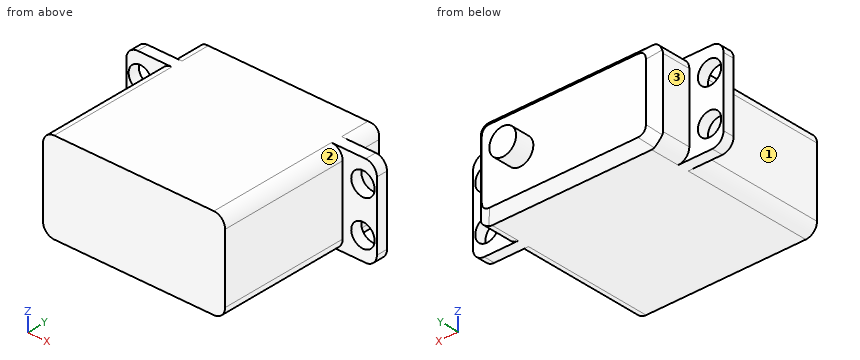
from build123d import *

# Parameters (mm, degrees)
BOSS_EXTRUDE1_DEPTH = 20.2
SKETCH2_R           = 2.975
BOSS_EXTRUDE2_DEPTH = 4.25
CUT_EXTRUDE1_START  = 29
SKETCH3_R           = 2.6
CUT_EXTRUDE1_DEPTH  = 4.25
CHAMFER1_SIZE       = 2
FILLET1_R           = 2.5


with BuildPart() as part:
    # Sketch1 → Boss-Extrude1 (new body)
    with BuildSketch(Plane.XY):
        Polygon((-20.25, 0), (20.25, 0), (20.25, 29), (27.85, 29), (27.85, 31.5), (20.25, 31.5), (20.25, 40), (-20.25, 40), (-20.25, 31.5), (-27.85, 31.5), (-27.85, 29), (-20.25, 29), align=None)
    extrude(amount=BOSS_EXTRUDE1_DEPTH)

    # Sketch2 → Boss-Extrude2 (add)
    with BuildSketch(Plane(origin=(0, 40, 0), x_dir=(1, 0, 0), z_dir=(0, 1, 0))):
        with Locations(Location((9.75, -10.1, 0), (0, 0, 90))):
            Circle(SKETCH2_R)
    extrude(amount=BOSS_EXTRUDE2_DEPTH)

    # Sketch3 → Cut-Extrude1 (cut)
    with BuildSketch(Plane(origin=(0, 0, 0), x_dir=(1, 0, 0), z_dir=(0, 1, 0)).offset(CUT_EXTRUDE1_START)):
        with Locations(Location((-24.75, -5.1, 0), (0, 0, 90))):
            Circle(SKETCH3_R)
        with Locations(Location((-24.75, -15.1, 0), (0, 0, 90))):
            Circle(SKETCH3_R)
    cut_extrude1 = extrude(amount=CUT_EXTRUDE1_DEPTH, mode=Mode.SUBTRACT)

    # Mirror1: Cut-Extrude1 across plane
    add(cut_extrude1.mirror(Plane(origin=(0, 0, 0), x_dir=(0, 0, 1), z_dir=(1, 0, 0))), mode=Mode.SUBTRACT)

    # Chamfer1
    chamfer1_edges = [part.edges().sort_by_distance(p)[0] for p in [
        (0, 40, 0),
        (0, 40, 20.2),
        (-20.25, 40, 10.1),
        (20.25, 40, 10.1),
    ]]
    chamfer(chamfer1_edges, length=CHAMFER1_SIZE)

    # Fillet1
    # the kernel refuses this fillet: 2.5 mm, written as the material it takes off along each edge
    with BuildSketch(Plane(origin=(20.25, -6.25, 0), x_dir=(-1, 0, 0), z_dir=(0, 1, 0)), Plane(origin=(-20.25, 29, 0), x_dir=(1, 0, 0), z_dir=(0, -1, 0)), Plane(origin=(-20.25, 29, 20.2), x_dir=(0, 0, -1), z_dir=(0, -1, 0)), Plane(origin=(20.25, -6.25, 20.2), x_dir=(0, 0, -1), z_dir=(0, 1, 0))) as fillet1_piece_1:
        with BuildLine():
            CenterArc((FILLET1_R, FILLET1_R), FILLET1_R, 180, 90)
            Line((0, FILLET1_R), (0, 0))
            Line((0, 0), (FILLET1_R, 0))
        make_face()
    extrude(amount=35.25, mode=Mode.SUBTRACT)
    with BuildSketch(Plane(origin=(20.25, -6.25, 0), x_dir=(-1, 0, 0), z_dir=(0, 1, 0))) as fillet1_piece_2_section:
        with BuildLine():
            CenterArc((FILLET1_R, FILLET1_R), FILLET1_R, 180, 90)
            Line((0, FILLET1_R), (0, 0))
            Line((0, 0), (FILLET1_R, 0))
        make_face()
    fillet1_piece_2 = extrude(amount=41.5, mode=Mode.PRIVATE)
    fillet1_piece_2 = split(fillet1_piece_2, bisect_by=Plane(origin=(19.684012214, 31.5, 0.565987786), z_dir=(0, 1, 0)), keep=Keep.TOP, mode=Mode.PRIVATE)
    add(fillet1_piece_2, mode=Mode.SUBTRACT)
    with BuildSketch(Plane(origin=(-20.25, 35.25, 0), x_dir=(1, 0, 0), z_dir=(0, -1, 0))) as fillet1_piece_3_section:
        with BuildLine():
            CenterArc((FILLET1_R, FILLET1_R), FILLET1_R, 180, 90)
            Line((0, FILLET1_R), (0, 0))
            Line((0, 0), (FILLET1_R, 0))
        make_face()
    fillet1_piece_3 = extrude(amount=41.5, mode=Mode.PRIVATE)
    fillet1_piece_3 = split(fillet1_piece_3, bisect_by=Plane(origin=(-19.684012214, 31.5, 0.565987786), z_dir=(0, 1, 0)), keep=Keep.TOP, mode=Mode.PRIVATE)
    add(fillet1_piece_3, mode=Mode.SUBTRACT)
    with BuildSketch(Plane(origin=(-27.85, 37.75, 0), x_dir=(1, 0, 0), z_dir=(0, -1, 0)), Plane(origin=(27.85, 22.75, 0), x_dir=(-1, 0, 0), z_dir=(0, 1, 0)), Plane(origin=(-27.85, 37.75, 20.2), x_dir=(0, 0, -1), z_dir=(0, -1, 0)), Plane(origin=(27.85, 22.75, 20.2), x_dir=(0, 0, -1), z_dir=(0, 1, 0))) as fillet1_piece_4:
        with BuildLine():
            CenterArc((FILLET1_R, FILLET1_R), FILLET1_R, 180, 90)
            Line((0, FILLET1_R), (0, 0))
            Line((0, 0), (FILLET1_R, 0))
        make_face()
    extrude(amount=15, mode=Mode.SUBTRACT)
    with BuildSketch(Plane(origin=(20.25, 25.25, 0), x_dir=(-1, 0, 0), z_dir=(0, 1, 0))) as fillet1_piece_5_section:
        with BuildLine():
            CenterArc((FILLET1_R, FILLET1_R), FILLET1_R, 180, 90)
            Line((0, FILLET1_R), (0, 0))
            Line((0, 0), (FILLET1_R, 0))
        make_face()
    fillet1_piece_5 = extrude(amount=19, mode=Mode.PRIVATE)
    fillet1_piece_5 = split(fillet1_piece_5, bisect_by=Plane(origin=(19.684012214, 29, 0.565987786), z_dir=(0, -1, 0)), keep=Keep.TOP, mode=Mode.PRIVATE)
    add(fillet1_piece_5, mode=Mode.SUBTRACT)
    with BuildSketch(Plane(origin=(20.25, 31.5, 0), x_dir=(-1, 0, 0), z_dir=(0, 1, 0)), Plane(origin=(20.25, 31.5, 20.2), x_dir=(0, 0, -1), z_dir=(0, 1, 0)), Plane(origin=(-20.25, 44.25, 20.2), x_dir=(0, 0, -1), z_dir=(0, -1, 0)), Plane(origin=(-20.25, 44.25, 0), x_dir=(1, 0, 0), z_dir=(0, -1, 0))) as fillet1_piece_6:
        with BuildLine():
            CenterArc((FILLET1_R, FILLET1_R), FILLET1_R, 180, 90)
            Line((0, FILLET1_R), (0, 0))
            Line((0, 0), (FILLET1_R, 0))
        make_face()
    extrude(amount=12.75, mode=Mode.SUBTRACT)
    with BuildSketch(Plane(origin=(20.25, 25.25, 20.2), x_dir=(0, 0, -1), z_dir=(0, 1, 0))) as fillet1_piece_7_section:
        with BuildLine():
            CenterArc((FILLET1_R, FILLET1_R), FILLET1_R, 180, 90)
            Line((0, FILLET1_R), (0, 0))
            Line((0, 0), (FILLET1_R, 0))
        make_face()
    fillet1_piece_7 = extrude(amount=19, mode=Mode.PRIVATE)
    fillet1_piece_7 = split(fillet1_piece_7, bisect_by=Plane(origin=(19.684012214, 29, 19.634012214), z_dir=(0, -1, 0)), keep=Keep.TOP, mode=Mode.PRIVATE)
    add(fillet1_piece_7, mode=Mode.SUBTRACT)
    with BuildSketch(Plane(origin=(-20.25, 35.25, 20.2), x_dir=(0, 0, -1), z_dir=(0, -1, 0))) as fillet1_piece_8_section:
        with BuildLine():
            CenterArc((FILLET1_R, FILLET1_R), FILLET1_R, 180, 90)
            Line((0, FILLET1_R), (0, 0))
            Line((0, 0), (FILLET1_R, 0))
        make_face()
    fillet1_piece_8 = extrude(amount=41.5, mode=Mode.PRIVATE)
    fillet1_piece_8 = split(fillet1_piece_8, bisect_by=Plane(origin=(-19.684012214, 31.5, 19.634012214), z_dir=(0, 1, 0)), keep=Keep.TOP, mode=Mode.PRIVATE)
    add(fillet1_piece_8, mode=Mode.SUBTRACT)
    with BuildSketch(Plane(origin=(20.25, -6.25, 20.2), x_dir=(0, 0, -1), z_dir=(0, 1, 0))) as fillet1_piece_9_section:
        with BuildLine():
            CenterArc((FILLET1_R, FILLET1_R), FILLET1_R, 180, 90)
            Line((0, FILLET1_R), (0, 0))
            Line((0, 0), (FILLET1_R, 0))
        make_face()
    fillet1_piece_9 = extrude(amount=41.5, mode=Mode.PRIVATE)
    fillet1_piece_9 = split(fillet1_piece_9, bisect_by=Plane(origin=(19.684012214, 31.5, 19.634012214), z_dir=(0, 1, 0)), keep=Keep.TOP, mode=Mode.PRIVATE)
    add(fillet1_piece_9, mode=Mode.SUBTRACT)
    with BuildSketch(Plane(origin=(-20.25, 44.25, 20.2), x_dir=(0, 0, -1), z_dir=(0, -1, 0))) as fillet1_piece_10_section:
        with BuildLine():
            CenterArc((FILLET1_R, FILLET1_R), FILLET1_R, 180, 90)
            Line((0, FILLET1_R), (0, 0))
            Line((0, 0), (FILLET1_R, 0))
        make_face()
    fillet1_piece_10 = extrude(amount=19, mode=Mode.PRIVATE)
    fillet1_piece_10 = split(fillet1_piece_10, bisect_by=Plane(origin=(-19.684012214, 29, 19.634012214), z_dir=(0, -1, 0)), keep=Keep.TOP, mode=Mode.PRIVATE)
    add(fillet1_piece_10, mode=Mode.SUBTRACT)
    with BuildSketch(Plane(origin=(-20.25, 44.25, 0), x_dir=(1, 0, 0), z_dir=(0, -1, 0))) as fillet1_piece_11_section:
        with BuildLine():
            CenterArc((FILLET1_R, FILLET1_R), FILLET1_R, 180, 90)
            Line((0, FILLET1_R), (0, 0))
            Line((0, 0), (FILLET1_R, 0))
        make_face()
    fillet1_piece_11 = extrude(amount=19, mode=Mode.PRIVATE)
    fillet1_piece_11 = split(fillet1_piece_11, bisect_by=Plane(origin=(-19.684012214, 29, 0.565987786), z_dir=(0, -1, 0)), keep=Keep.TOP, mode=Mode.PRIVATE)
    add(fillet1_piece_11, mode=Mode.SUBTRACT)
    with BuildSketch(Plane(origin=(22.333333333, 35.916666667, -2.083333333), x_dir=(-0.816496580927726, -0.4082482904638627, -0.4082482904638633), z_dir=(-0.5773502691896258, 0.5773502691896258, 0.5773502691896258)), Plane(origin=(22.333333333, 35.916666667, 22.283333333), x_dir=(0.40824829046386174, -0.4082482904638642, -0.8164965809277261), z_dir=(-0.5773502691896258, 0.5773502691896258, -0.5773502691896258))) as fillet1_piece_12:
        with BuildLine():
            CenterArc((FILLET1_R * 0.57735026919, FILLET1_R), FILLET1_R, 210, 60)
            Line((-FILLET1_R * 0.288675134595, FILLET1_R * 0.5), (0, 0))
            Line((0, 0), (FILLET1_R * 0.57735026919, 0))
        make_face()
    extrude(amount=10.68097998, mode=Mode.SUBTRACT)
    with BuildSketch(Plane(origin=(-22.333333333, 35.916666667, -2.083333333), x_dir=(0.8164965809277259, -0.4082482904638622, -0.40824829046386374), z_dir=(0.5773502691896258, 0.5773502691896258, 0.5773502691896258)), Plane(origin=(-22.333333333, 35.916666667, 22.283333333), x_dir=(-0.40824829046386424, -0.4082482904638618, -0.816496580927726), z_dir=(0.5773502691896258, 0.5773502691896258, -0.5773502691896258))) as fillet1_piece_13:
        with BuildLine():
            CenterArc((FILLET1_R * 0.57735026919, -FILLET1_R), FILLET1_R, 90, 60)
            Line((-FILLET1_R * 0.288675134595, -FILLET1_R * 0.5), (0, 0))
            Line((0, 0), (FILLET1_R * 0.57735026919, 0))
        make_face()
    extrude(amount=10.68097998, mode=Mode.SUBTRACT)


solid = part.part
For this review, take the finished solid that the model builds, in its own axes (mm). Face numbers are marked on the shaded views. A direction names the side the tool comes from. Round coordinates to 2 decimals unless told otherwise and drop trailing zeros. Loops run counter-clockwise (first coordinate to the right, second up) from the corner with the lowest first, then second, coordinate; pieces in that order, holes last. Notation, with made-up numbers: (-2, -6) - (18, -6) arc R25 ccw to (18, 32) - close; hole circle Ø6 at (-13.5, 64.5). An arc over 180 degrees is marked (long way). One line per question, with ' | ' between items.
Q1. Take a section at A-A (x = -24.75). Give the boundary of the cut face in (y, z).
Taken from the geometry:
outline: (29, 0) - (31.5, 0) - (31.5, 2.5) - (29, 2.5) - close; (29, 7.7) - (31.5, 7.7) - (31.5, 12.5) - (29, 12.5) - close; (29, 17.7) - (31.5, 17.7) - (31.5, 20.2) - (29, 20.2) - close
Q2. Take a section at D-D (z = 10.1). Give the boundary of the cut face in (x, y) (3 decimals), and give its area (3 significant figures).
Taken from the geometry:
outline: (-27.85, 29) - (-20.25, 29) - (-20.25, 0) - (20.25, 0) - (20.25, 29) - (27.85, 29) - (27.85, 31.5) - (20.25, 31.5) - (20.25, 38) - (18.25, 40) - (12.725, 40) - (12.725, 44.25) - (6.775, 44.25) - (6.775, 40) - (-18.25, 40) - (-20.25, 38) - (-20.25, 31.5) - (-27.85, 31.5) - close | area: 1,680 mm²
Q3. Tool access review of the marked faces 1, 2 and 3: name each direction out of +Z, -Z, +X, -X, +Y, -Y from which nothing blocks a thin tool from reaching the whole face with its end or side.
Taken from the geometry:
face 1: +Z, -Z, -X, -Y | face 2: +Z, +X, -Y | face 3: +Z, -Z, -X, +Y
Q4. For line 1 along X through (y, z) = (30.4, 5.1); line 2 along Z through (x, y) = (25, 31); line 3 along Z through (x, y) = (24, 30), list the stretches that pass through material, from the lowest coordinate up. Write a range as [from, to].
Taken from the geometry:
line 1: x = [-27.85, -27.35], [-22.15, 22.15], [27.35, 27.85] | line 2: z = [0, 2.51], [7.69, 12.51], [17.69, 20.2] | line 3: z = [0, 2.61], [7.59, 12.61], [17.59, 20.2]
Q5. Take a section at C-C (y = 5). Give the boundary of the cut face in (x, z), and give its area (3 significant figures).
Taken from the geometry:
outline: (-20.25, 2.5) arc R2.5 ccw to (-17.75, 0) - (17.75, 0) arc R2.5 ccw to (20.25, 2.5) - (20.25, 17.7) arc R2.5 ccw to (17.75, 20.2) - (-17.75, 20.2) arc R2.5 ccw to (-20.25, 17.7) - close | area: 813 mm²
Q6. Take a section at B-B (z = 5.1). Give the boundary of the cut face in (x, y).
Taken from the geometry:
outline: (-27.85, 29) - (-27.35, 29) - (-27.35, 31.5) - (-27.85, 31.5) - close; (-22.15, 29) - (-20.25, 29) - (-20.25, 0) - (20.25, 0) - (20.25, 29) - (22.15, 29) - (22.15, 31.5) - (20.25, 31.5) - (20.25, 38) - (18.25, 40) - (-18.25, 40) - (-20.25, 38) - (-20.25, 31.5) - (-22.15, 31.5) - close; (27.35, 29) - (27.85, 29) - (27.85, 31.5) - (27.35, 31.5) - close
Q7. For pin 1 (5 mm diameter, centred on x = 22.5, z = 11.5, fed in from +Y); pin 2 (1.5 mm diameter, centred on y = 25.5, z = 15, fed in from +X); pin 3 (2 mm diameter, centred on y = 33.5, z = 13.5, fed in from -X); pin 4 (10 mm diameter, centred on x = 21.5, y = 17, fed in from -Z), all flat-tipped, find the tip position at first contact; note any pin that passes through.
Taken from the geometry:
pin 1: stops at y = 38.25 | pin 2: stops at x = 20.25 | pin 3: stops at x = -20.25 | pin 4: stops at z = 0
